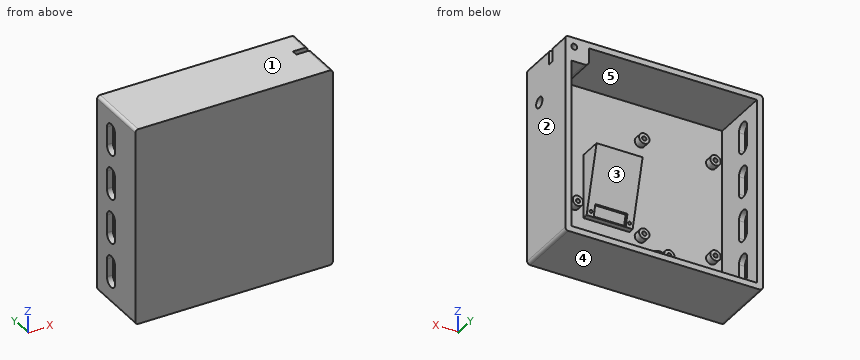
Autodesk Inventor part; units mm, degrees
ref_plane "YZ Plane" through (0, 0, 0) normal (1, 0, 0) x (0, 1, 0)
ref_plane "XZ Plane" through (0, 0, 0) normal (0, 1, 0) x (-1, 0, 0)
ref_plane "XY Plane" through (0, 0, 0) normal (0, 0, 1) x (1, 0, 0)
sketch "Esboço1" plane through (0, 0, 0) normal (0, 1, 0) x (-1, 0, 0)
  line L0 (-62.5, 62.5) -> (62.5, 62.5)
  line L1 (62.5, 62.5) -> (62.5, -62.5)
  line L2 (62.5, -62.5) -> (-62.5, -62.5)
  line L3 (-62.5, -62.5) -> (-62.5, 62.5)
  line L4 (-62.5, 62.5) -> (62.5, -62.5) construction
  line L5 (62.5, 62.5) -> (-62.5, -62.5) construction
  point P0 (0, 0)
  dimension "d0" = 125
  dimension "d1" = 125
extrude "Extrusão1" add sketch "Esboço1" along normal blind 4
sketch "Esboço2" plane through (0, 4, 0) normal (0, 1, 0) x (1, 0, 0)
  line L0 (-57.5, 55.5) -> (-21.5, 55.5)
  line L1 (-21.5, 55.5) -> (-21.5, 34.5)
  line L2 (-21.5, 34.5) -> (-57.5, 34.5)
  line L3 (-57.5, 34.5) -> (-57.5, 55.5)
  line L4 (62.5, 62.5) -> (-62.5, 62.5)
  line L5 (-62.5, 62.5) -> (-62.5, -62.5)
  circle A0 centre (-55, 53) radius 1.4
  circle A1 centre (-24, 37) radius 1.4
  circle A2 centre (-55, 53) radius 3.5
  circle A3 centre (-24, 37) radius 3.5
  line L6 (-57.6, 29.9977) -> (-4.6, 29.9977)
  line L7 (-4.6, 29.9977) -> (-4.6, -40.0023)
  line L8 (-4.6, -40.0023) -> (-57.6, -40.0023)
  line L9 (-57.6, -40.0023) -> (-57.6, 29.9977)
  circle A4 centre (-55.1, 27.4977) radius 1.45
  circle A5 centre (-55.1, -37.5023) radius 1.45
  circle A6 centre (-7.1, -37.5023) radius 1.45
  circle A7 centre (-7.1, 27.4977) radius 1.45
  circle A8 centre (-55.1, 27.4977) radius 3.5
  circle A9 centre (-7.1, 27.4977) radius 3.5
  circle A10 centre (-7.1, -37.5023) radius 3.5
  circle A11 centre (-55.1, -37.5023) radius 3.5
  line L10 (-1, 31) -> (27, 59) construction
  line L11 (27, 31) -> (-1, 59) construction
  line L12 (56, 55.5) -> (35, 55.5)
  line L13 (35, 55.5) -> (35, 12.5)
  line L14 (35, 12.5) -> (56, 12.5)
  line L15 (56, 12.5) -> (56, 55.5)
  circle A12 centre (53.5, 49) radius 1.4
  circle A13 centre (37.5, 19) radius 1.4
  line L16 (62.5, -62.5) -> (62.5, 62.5)
  circle A14 centre (53.5, 49) radius 3.5
  circle A15 centre (37.5, 19) radius 3.5
  line L17 (-62.5, -62.5) -> (62.5, -62.5)
  circle A16 centre (-11.5, 50.5) radius 2
  circle A17 centre (-11.5, 50.5) radius 3.5
  line L18 (-11.5, 54.6208) -> (-7.9313, 52.5604)
  line L19 (-7.9313, 52.5604) -> (-7.9313, 48.4396)
  line L20 (-7.9313, 48.4396) -> (-11.5, 46.3792)
  line L21 (-11.5, 46.3792) -> (-15.0687, 48.4396)
  line L22 (-15.0687, 48.4396) -> (-15.0687, 52.5604)
  line L23 (-15.0687, 52.5604) -> (-11.5, 54.6208)
  point P0 (0, 0)
  point P1 (13, 45)
  dimension "d7" = 5
  dimension "d9" = 2.8
  dimension "d10" = 2.5
  dimension "d11" = 2.5
  dimension "d12" = 2.5
  dimension "d13" = 2.5
  dimension "d14" = 7
  dimension "d15" = 7
  dimension "d16" = 53
  dimension "d17" = 70
  dimension "d18" = 2.9
  dimension "d19" = 2.9
  dimension "d20" = 2.9
  dimension "d21" = 2.9
  dimension "d22" = 48
  dimension "d23" = 2.5
  dimension "d25" = 48
  dimension "d26" = 2.5
  dimension "d27" = 65
  dimension "d28" = 2.5
  dimension "d29" = 7
  dimension "d30" = 7
  dimension "d31" = 7
  dimension "d32" = 7
  dimension "d39" = 21
  dimension "d40" = 43
  dimension "d41" = 2.8
  dimension "d42" = 2.8
  dimension "d43" = 7
  dimension "d44" = 6.5
  dimension "d45" = 6.5
  dimension "d46" = 2.5
  dimension "d47" = 6.5
  dimension "d48" = 2.5
  dimension "d49" = 7
  dimension "d50" = 7
  dimension "d51" = 2.8
  dimension "d57" = 36
  dimension "d58" = 21
  dimension "d83" = 22.4977
  dimension "d160" = 4
  dimension "d161" = 12
  dimension "d162" = 51
  dimension "d163" = 7
extrude "Extrusão2" add sketch "Esboço2" along normal blind 5 contours A2 L0 | L0 A2 L3 | L3 A2 | A3 L1 | L1 A3 L2 | L2 A3 | A8 L6 | L6 A8 L9 | L9 A8 | A9 L6 | L6 A9 L7 | A11 L8 L9 | L9 A11 | L7 A9 | A10 L7 | L7 A10 L8 | L8 A11 | L8 A10 | A14 L15 | L15 A14 | A15 L13 | L13 A15 picked at (-55.0563, 55.1299) picked at (-24.0563, 34.8701) picked at (-55.1583, 29.6442) picked at (-7.1583, 29.6442) picked at (-55.1583, -39.6488) picked at (-7.1583, -39.6488)
sketch "Esboço5" plane through (0, 9, 0) normal (0, 1, 0) x (1, 0, 0)
  circle A0 centre (29.5, 45) radius 1.45
  line L0 (29.5, 50) -> (27, 50)
  line L1 (25.5, 57.5) -> (25.5, 32.5)
  point P0 (0, 0)
  dimension "d70" = 2.9
  dimension "d71" = 5
  dimension "d72" = 4
extrude "Extrusão5" cut sketch "Esboço5" against normal blind 5
sketch "Esboço6" plane through (0, 4, 0) normal (0, 1, 0) x (1, 0, 0)
  line L0 (0, 26) -> (31, 26)
  line L1 (31, 26) -> (31, -17)
  line L2 (31, -17) -> (0, -17)
  line L3 (0, -17) -> (0, 26)
  line L4 (0, -17) -> (31, -17)
  line L5 (-1, 31) -> (27, 31)
  line L6 (-57.5, -40.0023) -> (-4.5, -40.0023)
  line L7 (-4.5, -40.0023) -> (-4.5, 29.9977)
  line L8 (-4.5, 29.9977) -> (-57.5, 29.9977)
  line L9 (-57.5, 29.9977) -> (-57.5, -40.0023)
  line L10 (-62.5, 62.5) -> (-62.5, -62.5)
  line L11 (-62.5, -62.5) -> (62.5, -62.5)
  line L12 (56, 12.5) -> (35, 12.5)
  line L13 (35, 12.5) -> (35, 55.5)
  line L14 (35, 55.5) -> (56, 55.5)
  line L15 (56, 55.5) -> (56, 12.5)
  line L16 (62.5, 62.5) -> (-62.5, 62.5)
  line L17 (62.5, -62.5) -> (62.5, 62.5)
  point P0 (0, 0)
  dimension "d76" = 43
  dimension "d78" = 5
  dimension "d79" = 53
  dimension "d80" = 70
  dimension "d81" = 5
  dimension "d82" = 22.4977
  dimension "d84" = 21
  dimension "d85" = 43
  dimension "d86" = 7
  dimension "d87" = 6.5
  dimension "d88" = 4.5
extrude "Extrusão6" add sketch "Esboço6" along normal blind 24 contours L0 L1 L2 L3
sketch "Esboço7" plane through (31, 4, 17) normal (1, 0, 0) x (0, 0, -1)
  line L0 (43.4351, 3.6251) -> (-38.6686, 25.6247)
  line L1 (-45.5, 0) -> (79.5, 0)
  line L2 (43.4351, 3.6251) -> (43.4351, 27.2402)
  line L3 (43.4351, 27.2402) -> (-38.6686, 25.6247)
  point P0 (17, -4)
  dimension "d92" = 85
  dimension "d93" = 15
extrude "Extrusão7" cut sketch "Esboço7" against normal blind 31
sketch "Esboço8" plane through (0, 19.2634, 17) normal (0, 0.9659, -0.2588) x (1, 0, 0)
  circle A0 centre (2.5, 41.5169) radius 0.95
  circle A1 centre (28.5, 41.5169) radius 0.95
  line L0 (0, 44.5169) -> (31, 44.5169)
  line L1 (0, 0) -> (0, 44.5169)
  line L2 (31, 44.5169) -> (31, 0)
  point P0 (0, 21.4065)
  dimension "d96" = 1.9
  dimension "d97" = 1.9
  dimension "d98" = 3
  dimension "d99" = 2.5
  dimension "d100" = 3
  dimension "d101" = 2.5
extrude "Extrusão8" cut sketch "Esboço8" against normal blind 4
ref_plane "Plano de trabalho2" through (2.5, 8.0976, -23.2575) normal (0, 0.9659, -0.2588) x (1, 0, 0)
sketch "Esboço10" plane through (2.5, 8.0976, -23.2575) normal (0, 0.9659, -0.2588) x (1, 0, 0)
  line L0 (2.2, -5.4) -> (23.8, -5.4)
  line L1 (23.8, -5.4) -> (23.8, 2.3)
  line L2 (23.8, 2.3) -> (2.2, 2.3)
  line L3 (2.2, 2.3) -> (2.2, -5.4)
  line L4 (-2.5, -41.5169) -> (-2.5, 3)
  line L5 (28.5, 3) -> (28.5, -41.5169)
  line L6 (-2.5, 3) -> (28.5, 3)
  point P0 (-2.5, -20.3692)
  dimension "d108" = 4.7
  dimension "d109" = 4.7
  dimension "d110" = 0.7
  dimension "d111" = 7.7
extrude "Extrusão10" cut sketch "Esboço10" along normal mid plane 3.7
sketch "Esboço11" plane through (0, 0, 0) normal (0, -1, 0) x (1, 0, 0)
  line L0 (-66.5, -66.5) -> (66.5, -66.5)
  line L1 (66.5, -66.5) -> (66.5, 66.5)
  line L2 (66.5, 66.5) -> (-66.5, 66.5)
  line L3 (-66.5, 66.5) -> (-66.5, -66.5)
  line L4 (-66.5, -66.5) -> (66.5, 66.5) construction
  line L5 (66.5, -66.5) -> (-66.5, 66.5) construction
  line L6 (62.5, 62.5) -> (62.5, -62.5)
  line L7 (-62.5, -62.5) -> (62.5, -62.5)
  line L8 (62.5, -62.5) -> (62.5, 62.5)
  line L9 (62.5, 62.5) -> (-62.5, 62.5)
  line L10 (-62.5, 62.5) -> (-62.5, -62.5)
  line L11 (-62.5, -62.5) -> (62.5, 62.5) construction
  line L12 (62.5, -62.5) -> (-62.5, 62.5) construction
  point P0 (0, 0)
  dimension "d114" = 133
  dimension "d115" = 133
extrude "Extrusão11" add sketch "Esboço11" against normal blind 44
fillet "Arredondamento2" radius 2 4 edges at (-66.5, 22, 66.5) (66.5, 22, 66.5) (66.5, 22, -66.5) (-66.5, 22, -66.5)
sketch "Esboço13" plane through (-66.5, 0, -64.5) normal (-1, 0, 0) x (0, 0, 1)
  arc A0 (13.41, 32.65) -> (13.41, 23.35) centre (13.41, 28) ccw
  line L0 (0, 44) -> (129, 44)
  arc A1 (25.41, 23.35) -> (25.41, 32.65) centre (25.41, 28) ccw
  line L1 (13.41, 32.65) -> (25.41, 32.65)
  line L2 (25.41, 23.35) -> (13.41, 23.35)
  arc A2 (43.47, 32.65) -> (43.47, 23.35) centre (43.47, 28) ccw
  arc A3 (55.47, 23.35) -> (55.47, 32.65) centre (55.47, 28) ccw
  line L3 (43.47, 32.65) -> (55.47, 32.65)
  line L4 (55.47, 23.35) -> (43.47, 23.35)
  arc A4 (73.53, 32.65) -> (73.53, 23.35) centre (73.53, 28) ccw
  arc A5 (85.53, 23.35) -> (85.53, 32.65) centre (85.53, 28) ccw
  line L5 (73.53, 32.65) -> (85.53, 32.65)
  line L6 (85.53, 23.35) -> (73.53, 23.35)
  arc A6 (103.59, 32.65) -> (103.59, 23.35) centre (103.59, 28) ccw
  arc A7 (115.59, 23.35) -> (115.59, 32.65) centre (115.59, 28) ccw
  line L7 (103.59, 32.65) -> (115.59, 32.65)
  line L8 (115.59, 23.35) -> (103.59, 23.35)
  line L9 (131, 0) -> (131, 44)
  line L10 (-2, 44) -> (-2, 0)
  line L11 (129, 44) -> (129, 0)
  line L12 (0, 0) -> (0, 44)
  point P0 (64.5, 0)
  dimension "d131" = 9.3
  dimension "d132" = 16
  dimension "d133" = 9.3
  dimension "d134" = 12
  dimension "d135" = 9.3
  dimension "d136" = 9.3
  dimension "d137" = 12
  dimension "d138" = 9.3
  dimension "d139" = 9.3
  dimension "d140" = 12
  dimension "d141" = 9.3
  dimension "d142" = 9.3
  dimension "d143" = 12
  dimension "d145" = 16
  dimension "d146" = 16
  dimension "d147" = 16
  dimension "d150" = 13.41
  dimension "d151" = 18.06
  dimension "d152" = 18.06
  dimension "d153" = 18.06
extrude "Extrusão12" cut sketch "Esboço13" against normal blind 5
sketch "Esboço15" plane through (0, 44, 0) normal (0, 1, 0) x (1, 0, 0)
  circle A0 centre (-11.5, 50.5) radius 2
  line L0 (-62.5, 62.5) -> (62.5, 62.5)
  line L1 (-62.5, -62.5) -> (-62.5, 62.5)
  line L2 (-11.5, 54.7301) -> (-7.8366, 52.6151)
  line L3 (-7.8366, 52.6151) -> (-7.8366, 48.3849)
  line L4 (-7.8366, 48.3849) -> (-11.5, 46.2699)
  line L5 (-11.5, 46.2699) -> (-15.1634, 48.3849)
  line L6 (-15.1634, 48.3849) -> (-15.1634, 52.6151)
  line L7 (-15.1634, 52.6151) -> (-11.5, 54.7301)
  circle A1 centre (-11.5, 50.5) radius 7
  point P0 (0, 0)
  point P1 (56, 62.5)
  dimension "d164" = 4
  dimension "d165" = 12
  dimension "d166" = 51
  dimension "d168" = 14
extrude "Extrusão14" add sketch "Esboço15" against normal blind 40 contours A1
sketch "Esboço18" plane through (-62.5, 4, -62.5) normal (0, 0, 1) x (1, 0, 0)
  line L0 (125, 40) -> (0, 40)
  line L1 (43.5378, 40) -> (60.5378, 40)
  line L2 (60.5378, 40) -> (60.5378, 10)
  line L3 (60.5378, 10) -> (43.5378, 10)
  line L4 (43.5378, 10) -> (43.5378, 40)
  point P0 (62.5, -4)
  dimension "d179" = 30
  dimension "d182" = 17
extrude "Extrusão16" cut sketch "Esboço18" along normal blind 20.7
sketch "Esboço19" plane through (0, 4, 0) normal (0, 1, 0) x (1, 0, 0)
  line L0 (-11.5, 54.7301) -> (-7.8366, 52.6151)
  line L1 (-7.8366, 52.6151) -> (-7.8366, 48.3849)
  line L2 (-7.8366, 48.3849) -> (-11.5, 46.2699)
  line L3 (-11.5, 46.2699) -> (-15.1634, 48.3849)
  line L4 (-15.1634, 48.3849) -> (-15.1634, 52.6151)
  line L5 (-15.1634, 52.6151) -> (-11.5, 54.7301)
  point P0 (0, 0)
  point P1 (-11.5, 50.5)
extrude "Extrusão17" add sketch "Esboço19" along normal blind 5.9
sketch "Esboço20" plane through (-11.5, 14, -50.5) normal (0, 1, 0) x (1, 0, 0)
  circle A0 centre (0, 0) radius 7
  point P0 (11.5, -50.5)
extrude "Extrusão18" add sketch "Esboço20" along normal blind 5
sketch "Esboço21" plane through (-11.5, 19, -50.5) normal (0, 1, 0) x (1, 0, 0)
  circle A0 centre (0, 0) radius 2
  point P0 (11.5, -50.5)
  dimension "d187" = 4
extrude "Extrusão19" cut sketch "Esboço21" against normal blind 16
sketch "Esboço22" plane through (0, 44, 0) normal (0, 1, 0) x (1, 0, 0)
  line L0 (-62.5, -62.5) -> (62.5, -62.5)
  line L1 (62.5, -62.5) -> (50.5, -62.5)
  line L2 (50.5, -62.5) -> (50.5, -50.5)
  line L3 (50.5, -50.5) -> (62.5, -50.5)
  line L4 (62.5, -50.5) -> (62.5, -62.5)
  point P0 (0, 0)
  dimension "d192" = 12
  dimension "d193" = 12
extrude "Extrusão20" add sketch "Esboço22" against normal blind 40
fillet "Arredondamento3" radius 3 1 edges at (50.5, 24, 50.5)
sketch "Esboço24" plane through (-64.5, 0, 66.5) normal (0, 0, 1) x (1, 0, 0)
  line L0 (131, 44) -> (131, 0)
  line L1 (131, 29) -> (121, 29)
  line L2 (121, 29) -> (121, 25)
  line L3 (121, 25) -> (131, 25)
  line L4 (131, 25) -> (131, 29)
  line L5 (0, 44) -> (129, 44)
  point P0 (64.5, 0)
  dimension "d197" = 10
  dimension "d198" = 4
  dimension "d199" = 15
extrude "Extrusão21" cut sketch "Esboço24" against normal blind 10
sketch "Esboço25" plane through (0, 44, 0) normal (0, 1, 0) x (1, 0, 0)
  circle A0 centre (60.5, -60.5) radius 2.005
  line L0 (66.5, -64.5) -> (66.5, 64.5)
  line L1 (-64.5, -66.5) -> (64.5, -66.5)
  point P0 (0, 0)
  dimension "d202" = 4.01
  dimension "d203" = 6
  dimension "d204" = 6
extrude "Extrusão22" cut sketch "Esboço25" against normal blind 36.75
sketch "Esboço26" plane through (66.5, 0, 64.5) normal (1, 0, 0) x (0, 0, -1)
  circle A0 centre (28, 14) radius 3.6
  line L0 (129, 0) -> (0, 0)
  line L1 (-2, 25) -> (-2, 0)
  point P0 (64.5, 0)
  dimension "d207" = 7.2
  dimension "d208" = 14
  dimension "d209" = 30
extrude "Extrusão23" cut sketch "Esboço26" against normal blind 5
properties part number "Caixa"
Verification items for the finished model (mm, model axes). Face numbers are marked on the shaded views. A direction names the side the tool comes from. Coordinates: 2 decimals unless noted, no trailing zeros. Order: outer loops, then holes, each group sorted by start corner. A loop starts at its lowest first (then second) coordinate and runs counter-clockwise, first axis right, second up. Notation, with made-up numbers: M 41,-22 L 53,-22 A25 cw 53,4 Z; hole C 37.25,65 d6. An arc over 180 degrees is marked long. One line per item, written item: value. Start each with the question number.
Item 1: Sectioned sample at B-B on x = -36. Record the cut outline in (y, z).
Item 2: Access from +Z, -Z, +X, -X, +Y, -Y to the whole of each face (thin tool, end or side, straight path). Record for the marked faces 4 and 5.
Item 3: Thickness scan on probe 1 along X at (y, z) = (8, -5); probe 2 along Z at (x, y) = (53.5, 7.3); probe 3 along X at (y, z) = (6.2, -37). Record the ranges inside material, lowest first.
Item 4: Depth check by flat-ended pin: P1, Ø10, axis at x = -30, z = -41.5, coming from the +Y side; P2, Ø0.8, axis at x = -24, z = -37, coming from the +Y side; P3, Ø3.5, axis at x = -11.5, z = -50.5, coming from the +Y side. Enter the tip coordinate at first touch or a pass-through.
Item 5: Mould release check, pull along Z, two halves, no side actions. Record for the marked faces 1, 2 and 3: pulls with the +Z half, pulls with the -Z half, needs draft (parallel to the pull), parting line crosses it, or undercut.
Item 6: Sectioned sample at A-A on y = 21. Record the cut outline in (x, z) (3 decimals).
Calculated:
1. outline: M 0,-66.5 L 44,-66.5 L 44,-62.5 L 4,-62.5 L 4,62.5 L 44,62.5 L 44,66.5 L 0,66.5 Z
2. face 4: -Z, +X, -X, +Y, -Y
2. face 5: +Y
3. probe 1: -66.5 to -62.5, 0 to 31, 62.5 to 66.5
3. probe 2: -66.5 to -62.5, -52.5 to -50.4, -47.6 to -45.5, 50.5 to 66.5
3. probe 3: -66.5 to -62.5, -27.5 to -25.4, -22.6 to -20.5, 62.5 to 66.5
4. P1: y = 9
4. P2: y = 4
4. P3: y = 3
5. face 1: pulls with the +Z half
5. face 2: needs draft
5. face 3: undercut
6. outline: M -66.5,-64.5 A2 ccw -64.5,-66.5 L 64.5,-66.5 A2 ccw 66.5,-64.5 L 66.5,64.5 A2 ccw 64.5,66.5 L -64.5,66.5 A2 ccw -66.5,64.5 Z; hole M -62.5,-62.5 L 62.5,-62.5 L 62.5,50.5 L 53.5,50.5 A3 cw 50.5,53.5 L 50.5,62.5 L -62.5,62.5 Z; hole C 60.5,60.5 d4.01
